Read the model definition and answer for the solid it produces. Units are mm, in the model's axes. Face numbers are marked on the shaded views. Coordinates: 2 decimals unless noted, no trailing zeros. Write each loop counter-clockwise with the first axis right and the second up, starting at its lowest first coordinate (ties: lowest second). Pieces come first, ordered by that corner, then holes.
Item 1: Section C-C (z = 8) is taken. Give the vertices of the cut face in (x, y), then the cut area to 3 significant figures.
Item 2: Straight lines are drawn through the part: probe 1 along Y at (x, z) = (0, 18.25); probe 2 along X at (y, z) = (23, 24); probe 3 along X at (y, z) = (116, 15.75). For each, find the intervals that lie inside material, in ascending order.
Item 3: Section A-A (x = 0) is taken. Give the vertices of the cut face in (y, z).
Item 4: Determine the mould class of the marked faces 1 and 2 for opening direction Y: released by +Y, released by -Y, zero draft, split by the parting line, or undercut.
Item 5: Each of these flat-tipped pins is pushed along its axis until it touches: P1, Ø5, axis at x = -28, z = 13.5, coming from the +Y side; P2, Ø4, axis at y = -7.5, z = 15, coming from the -X side; P3, Ø4, axis at x = -91.5, z = 2.5, coming from the +Y side. Where does it stop, or does it pass through?
Autodesk Inventor part; units mm, degrees
ref_plane "YZ Plane" through (0, 0, 0) normal (1, 0, 0) x (0, 1, 0)
ref_plane "XZ Plane" through (0, 0, 0) normal (0, 1, 0) x (-1, 0, 0)
ref_plane "XY Plane" through (0, 0, 0) normal (0, 0, 1) x (1, 0, 0)
sketch "Sketch1" plane through (0, 0, 0) normal (0, 0, 1) x (1, 0, 0)
  circle A0 centre (0, 0) radius 161.1312
  circle A1 centre (0, 0) radius 151.6062
  circle A2 centre (0, 0) radius 153.1937
  circle A3 centre (0, 0) radius 159.5438
  dimension "d2" = 9.525
  dimension "d3" = 303.2125
  dimension "d4" = 322.2625
  dimension "d13" = 306.3875
  dimension "d14" = 319.0875
  dimension "d15" = 6.35
  dimension "d16" = 1.5875
  dimension "d21" = 0
extrude "Extrusion1" add sketch "Sketch1" along normal blind 1.5875 contours A3
extrude "Extrusion2" add sketch "Sketch1" along normal blind 25.4
properties part number "tubecap"
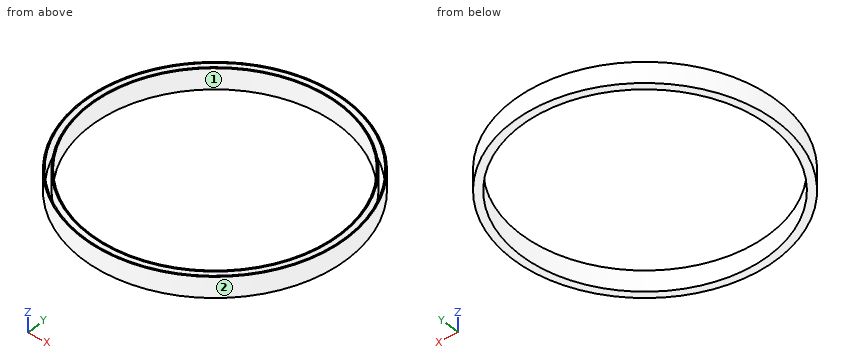
Established:
1. outline: circle Ø322.26 at (0, 0); circle Ø306.39 at (0, 0); hole circle Ø319.09 at (0, 0); hole circle Ø303.21 at (0, 0)
1. area: 3,120 mm2
2. probe 1: y = -161.13 to -159.54, -153.19 to -151.61, 151.61 to 153.19, 159.54 to 161.13
2. probe 2: x = -159.48 to -157.88, -151.46 to -149.85, 149.85 to 151.46, 157.88 to 159.48
2. probe 3: x = -111.84 to -109.54, -100.06 to -97.61, 97.61 to 100.06, 109.54 to 111.84
3. outline: (-161.13, 0) - (-151.61, 0) - (-151.61, 25.4) - (-153.19, 25.4) - (-153.19, 1.59) - (-159.54, 1.59) - (-159.54, 25.4) - (-161.13, 25.4) - close; (151.61, 0) - (161.13, 0) - (161.13, 25.4) - (159.54, 25.4) - (159.54, 1.59) - (153.19, 1.59) - (153.19, 25.4) - (151.61, 25.4) - close
4. face 1: undercut
4. face 2: split by the parting line
5. P1: stops at y = 159.1
5. P2: stops at x = -161.04
5. P3: stops at y = 133.99
